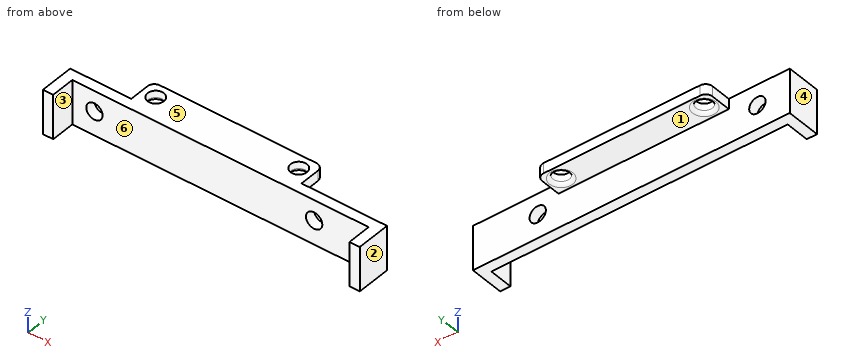
Autodesk Inventor part; units mm, degrees
ref_plane "YZ Plane" through (0, 0, 0) normal (1, 0, 0) x (0, 1, 0)
ref_plane "XZ Plane" through (0, 0, 0) normal (0, 1, 0) x (-1, 0, 0)
ref_plane "XY Plane" through (0, 0, 0) normal (0, 0, 1) x (1, 0, 0)
sketch "Sketch1" plane through (0, 0, 0) normal (0, 1, 0) x (-1, 0, 0)
  line L0 (0, 0) -> (93, 0)
  line L1 (93, 0) -> (93, -13)
  line L2 (93, -13) -> (0, -13)
  line L3 (0, -13) -> (0, 0)
  circle A0 centre (83.5, -6) radius 2.4
  circle A1 centre (19, -6) radius 2.4
  dimension "d0" = 93
  dimension "d1" = 13
  dimension "d2" = 4.8
  dimension "d3" = 4.8
  dimension "d4" = 6
  dimension "d5" = 6
  dimension "d6" = 19
  dimension "d7" = 9.5
extrude "Extrusion1" add sketch "Sketch1" along normal blind 3
sketch "Sketch2" plane through (0, 3, 0) normal (0, 1, 0) x (1, 0, 0)
  line L0 (-93, 0) -> (0, 0)
  line L1 (0, 13) -> (-93, 13)
  line L2 (0, 0) -> (-3, 0)
  line L3 (-3, 0) -> (-3, 13)
  line L4 (-3, 13) -> (0, 13)
  line L5 (0, 13) -> (0, 0)
  line L6 (-93, 0) -> (-90, 0)
  line L7 (-90, 0) -> (-90, 13)
  line L8 (-90, 13) -> (-93, 13)
  line L9 (-93, 13) -> (-93, 0)
  dimension "d10" = 3
  dimension "d11" = 3
extrude "Extrusion2" add sketch "Sketch2" against normal blind 10 contours L9 L1 L7 L0 | L3 L1 L5 L0
sketch "Sketch3" plane through (0, 3, 0) normal (0, 1, 0) x (1, 0, 0)
  line L0 (-3, 0) -> (-90, 0)
  line L1 (-75.0955, 0) -> (-25.0955, 0)
  line L2 (-25.0955, 0) -> (-25.0955, 3)
  line L3 (-25.0955, 3) -> (-75.0955, 3)
  line L4 (-75.0955, 3) -> (-75.0955, 0)
  point P0 (0, 0)
  dimension "d14" = 50
  dimension "d15" = 3
extrude "Extrusion3" add sketch "Sketch3" along normal blind 8
fillet "Fillet1" radius 2 2 edges at (-25.0955, 11, -1.5) (-75.0955, 11, -1.5)
sketch "Sketch4" plane through (-25.0955, 3, -3) normal (0, 0, -1) x (-1, 0, 0)
  circle A0 centre (46, 4) radius 2.4
  circle A1 centre (4, 4) radius 2.4
  line L0 (2, 8) -> (48, 8)
  line L1 (0, 0) -> (0, 6)
  line L2 (50, 0) -> (50, 6)
  point P0 (-25.0955, -3)
  dimension "d19" = 4.8
  dimension "d20" = 4.8
  dimension "d21" = 4
  dimension "d22" = 4
  dimension "d23" = 4
  dimension "d24" = 4
extrude "Extrusion4" cut sketch "Sketch4" against normal blind 8
fillet "Fillet2" radius 1 2 edges at (-68.6955, 7, -3) (-26.6955, 7, -3)
properties part number "PSUMount"
For this review, take the finished solid that the model builds, in its own axes (mm). Face numbers are marked on the shaded views. A direction names the side the tool comes from. Round coordinates to 2 decimals unless told otherwise and drop trailing zeros. Order: outer loops, then holes, each group sorted by start corner. A loop starts at its lowest first (then second) coordinate and runs counter-clockwise, first axis right, second up. Notation, with made-up numbers: (-27.75, 87.5) -> (28.25, 87.5) arc R21 cw to (28.25, 105.5) -> close; hole circle Ø10 at (59, 10.5). An arc over 180 degrees is marked (long way). Use a Markdown table: item, result.
Item 1: Take a section at C-C (x = -19). State the section outline as (y, z) points, plus the area to 3 significant figures.
Resolved:
| item | result |
|---|---|
| outline | (0, -13) -> (3, -13) -> (3, -8.4) -> (0, -8.4) -> close; (0, -3.6) -> (3, -3.6) -> (3, 0) -> (0, 0) -> close |
| area | 24.6 mm² |
Item 2: Take a section at A-A (z = -6). State the section outline as (x, y) points.
Resolved:
| item | result |
|---|---|
| outline | (-93, -7) -> (-90, -7) -> (-90, 0) -> (-85.9, 0) -> (-85.9, 3) -> (-93, 3) -> close; (-81.1, 0) -> (-21.4, 0) -> (-21.4, 3) -> (-81.1, 3) -> close; (-16.6, 0) -> (-3, 0) -> (-3, -7) -> (0, -7) -> (0, 3) -> (-16.6, 3) -> close |
Item 3: Machinability: for the marked faces 1 and 2, which of the approach directions +Z, -Z, +X, -X, +Y, -Y give a long, thin tool a straight path to every point of the face, cutting with its end or side? Answer none if there is none.
Resolved:
| item | result |
|---|---|
| face 1 | -Z, +X, -X, +Y |
| face 2 | +Z, -Z, +X, +Y, -Y |
Item 4: Draft analysis for pull direction X (two halves, no side actions). For the marked faces 3, 4, 5 and 6, state which applies: +X half, -X half, draft (parallel to the pull), parting line (faces both ways), or undercut.
Resolved:
| item | result |
|---|---|
| face 3 | undercut |
| face 4 | -X half |
| face 5 | draft |
| face 6 | undercut |
Item 5: Take a section at B-B (y = 7). State the section outline as (x, z) points, plus the area to 3 significant figures.
Resolved:
| item | result |
|---|---|
| outline | (-75.1, -3) -> (-74.5, -3) arc R1 ccw to (-73.5, -2) -> (-73.5, 0) -> (-75.1, 0) -> close; (-68.7, -2) arc R1 ccw to (-67.7, -3) -> (-32.5, -3) arc R1 ccw to (-31.5, -2) -> (-31.5, 0) -> (-68.7, 0) -> close; (-26.7, -2) arc R1 ccw to (-25.7, -3) -> (-25.1, -3) -> (-25.1, 0) -> (-26.7, 0) -> close |
| area | 120 mm² |
Item 6: For line 1 along Z through (x, y) = (-83.5, 1.4); line 2 along Y through (x, z) = (-39, -6.75); line 3 along Z through (x, y) = (-66.5, 9.25), list the stretches that pass through material, from the lowest coordinate up. Write a range as [from, to].
Resolved:
| item | result |
|---|---|
| line 1 | z = [-13, -8.4], [-3.6, 0] |
| line 2 | y = [0, 3] |
| line 3 | z = [-3, 0] |
Item 7: Take a section at D-D (y = -2). State the section outline as (x, z) points, plus the area to 3 significant figures.
Resolved:
| item | result |
|---|---|
| outline | (-93, -13) -> (-90, -13) -> (-90, 0) -> (-93, 0) -> close; (-3, -13) -> (0, -13) -> (0, 0) -> (-3, 0) -> close |
| area | 78.0 mm² |
Item 8: For pin 1 (6.5 mm diameter, centred on x = -43.5, z = -5, fed in from -Y); pin 2 (1 mm diameter, centred on x = -12.5, z = -7, fed in from +Y); pin 3 (3.5 mm diameter, centred on y = 7, z = -1.5, fed in from -X); pin 4 (4 mm diameter, centred on x = -71.1, y = 7, fed in from +Z), all flat-tipped, find the tip position at first contact; note any pin that passes through.
Resolved:
| item | result |
|---|---|
| pin 1 | stops at y = 0 |
| pin 2 | stops at y = 3 |
| pin 3 | stops at x = -75.1 |
| pin 4 | passes through |
